```python
from build123d import *

# Parameters (mm, degrees)
EXTRUDE_1_DEPTH     = 5
EXTRUDE_7_DEPTH     = 2.220844282
CUT_EXTRUDE_5_DEPTH = 4.5
SKETCH_22_W         = 3
SKETCH_22_H         = 6
CUT_EXTRUDE_7_DEPTH = 10
SKETCH_24_W         = 3
SKETCH_24_H         = 6
CUT_EXTRUDE_8_DEPTH = 2
SKETCH_25_W         = 3
SKETCH_25_H         = 6
CUT_EXTRUDE_9_DEPTH = 2


with BuildPart() as part:
    # 草圖1 → 填料-伸長1 (new, symmetric)
    with BuildSketch(Plane.XY):
        with BuildLine():
            Line((0, 0), (0, -20))
            ThreePointArc((0, -20), (4.217076995, -21.746770485), (8.434153991, -20))
            Line((8.434153991, -20), (8.434153991, 0))
            ThreePointArc((8.434153991, 0), (4.217076995, 1.305083655), (0, 0))
        make_face()
    extrude(amount=EXTRUDE_1_DEPTH, both=True)

    # 草圖19 → 填料-伸長7 (add, symmetric)
    with BuildSketch(Plane(origin=(-5.031859453, -10, 0), x_dir=(1, 0, 0), z_dir=(0, 1, 0))):
        with BuildLine():
            Line((8.364623855, 4.848181061), (19.186976182, 4.848181061))
            ThreePointArc((19.186976182, 4.848181061), (24.038353521, -0.003196277), (19.186976182, -4.854573616))
            Line((19.186976182, -4.854573616), (8.364623855, -4.854573616))
            Line((8.364623855, -4.854573616), (8.364623855, 4.848181061))
        make_face()
    extrude(amount=EXTRUDE_7_DEPTH, both=True)

    # 草圖21 → 除料-伸長5 (cut)
    with BuildSketch(Plane(origin=(0, -7.779155718, 0), x_dir=(1, 0, 0), z_dir=(0, 1, 0))):
        with BuildLine():
            Line((8.434153991, 3.848181061), (14.041459842, 3.848181061))
            ThreePointArc((14.041459842, 3.848181061), (17.892837181, -0.003196277), (14.041459842, -3.854573616))
            Line((14.041459842, -3.854573616), (8.434153991, -3.854573616))
            Line((8.434153991, -3.854573616), (8.434153991, 3.848181061))
        make_face()
    extrude(amount=-CUT_EXTRUDE_5_DEPTH, mode=Mode.SUBTRACT)

    # 草圖22 → 除料-伸長7 (cut)
    with BuildSketch(Plane.XY.offset(5)):
        with Locations((4.5, -10.185420111)):
            Rectangle(SKETCH_22_W, SKETCH_22_H)
    extrude(amount=-CUT_EXTRUDE_7_DEPTH, mode=Mode.SUBTRACT)

    # 草圖24 → 除料-伸長8 (cut)
    with BuildSketch(Plane(origin=(0, 0, -5), x_dir=(-1, 0, 0), z_dir=(0, 0, -1))):
        with Locations((-1.5, -10.185420111)):
            Rectangle(SKETCH_24_W, SKETCH_24_H)
    extrude(amount=-CUT_EXTRUDE_8_DEPTH, mode=Mode.SUBTRACT)

    # 草圖25 → 除料-伸長9 (cut)
    with BuildSketch(Plane.XY.offset(5)):
        with Locations((1.5, -10.185420111)):
            Rectangle(SKETCH_25_W, SKETCH_25_H)
    extrude(amount=-CUT_EXTRUDE_9_DEPTH, mode=Mode.SUBTRACT)


solid = part.part
```
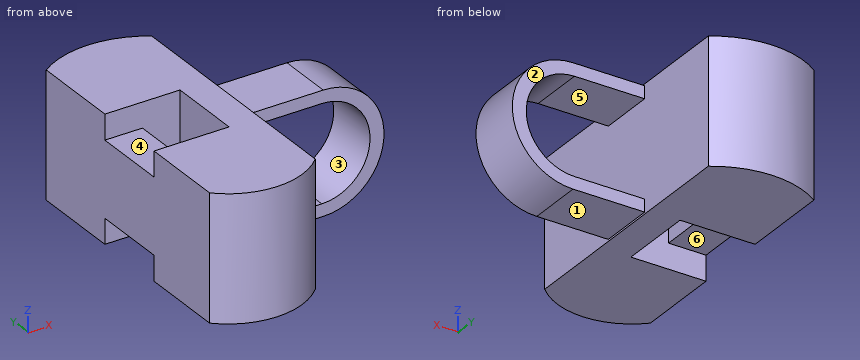
Input: part model. Units: mm. Frame: model coordinates. Face numbers are marked on the shaded views. A direction names the side the tool comes from. Coordinates: 2 decimals unless noted, no trailing zeros. Loops run counter-clockwise (first coordinate to the right, second up) from the corner with the lowest first, then second, coordinate; pieces in that order, holes last. Notation, with made-up numbers: M 83.5,-27 L 115.5,-27 A28 ccw 115.5,-4 Z; hole C 34,76.25 d9. An arc over 180 degrees is marked long. Use a Markdown table: item, result. Add a question column.
1) Set-up query: the marked faces 4, 5 and 6. Return all of +Z, -Z, +X, -X, +Y, -Y with unobstructed straight access to the full face (end or side cutting, diameter ignored); none if empty.
2) Section B-B, the plane z = 0.75. Return the cut outline in (x, y), plus the area to 3 significant figures.
3) Draft query along Z for the marked faces 1, 2 and 3. Return one class per face: +Z half, -Z half, draft (parallel to the pull), parting line (faces both ways), or undercut.
4) Line query: L1, parallel to X at y = -11.5, z = 0; L2, parallel to X at y = -10, z = -2.5; L3, parallel to Y at x = 4, z = 2.5. Output: solid intervals per line, ascending. Write a range as from..to.
5) Section C-C, the plane x = 16. Return the cut outline in (y, z), plus the area to 3 significant figures.
6) Section D-D, the plane z = -3.5. Return the cut outline in (x, y), plus the area to 3 significant figures.
7) Pin query (flat end, axial travel): P1, Ø3, axis at x = 12, z = -1, coming from the -Y side; P2, Ø5, axis at y = -13.5, z = -2.5, coming from the +X side; P3, Ø2.5, axis at x = 2, y = -11.5, coming from the +Z side; P4, Ø3.5, axis at x = 10.5, y = -9.5, coming from the -Z side. Return the tip coordinate at first contact, or that it passes through.
8) Section A-A, the plane y = -11.75. Return the cut outline in (x, z).
Answer below:
| question | item | result |
|---|---|---|
| 1 | face 4 | +Z, -X |
| 1 | face 5 | +Y, -Y |
| 1 | face 6 | -Z, -X |
| 2 | outline | M 0,-20 A5.96 ccw 8.43,-20 L 8.43,0 A7.47 ccw 0,0 Z; M 17.82,-12.22 L 18.95,-12.22 L 18.95,-7.78 L 17.82,-7.78 Z; hole M 3,-13.19 L 6,-13.19 L 6,-7.19 L 3,-7.19 Z |
| 2 | area | 173 mm2 |
| 3 | face 1 | -Z half |
| 3 | face 2 | draft |
| 3 | face 3 | undercut |
| 4 | L1 | 0..3, 6..8.43, 17.89..19.01 |
| 4 | L2 | 0..3, 6..8.43, 16.97..18.31 |
| 4 | L3 | -21.74..-13.19, -7.19..1.3 |
| 5 | outline | M -12.22,-4.48 L -7.78,-4.48 L -7.78,-3.31 L -12.22,-3.31 Z; M -12.22,3.32 L -7.78,3.32 L -7.78,4.49 L -12.22,4.49 Z |
| 5 | area | 10.4 mm2 |
| 6 | outline | M 0,-20 A5.96 ccw 8.43,-20 L 8.43,0 A7.47 ccw 0,0 L 0,-7.19 L 6,-7.19 L 6,-13.19 L 0,-13.19 Z; M 15.64,-12.22 L 17.51,-12.22 L 17.51,-7.78 L 15.64,-7.78 Z |
| 6 | area | 159 mm2 |
| 7 | P1 | through |
| 7 | P2 | x = 18.99 |
| 7 | P3 | z = 3 |
| 7 | P4 | z = -4.85 |
| 8 | outline | M 0,-3 L 3,-3 L 3,3 L 0,3 Z; M 6,-5 L 8.43,-5 L 8.43,-4.85 L 14.16,-4.85 A4.85 ccw 14.16,4.85 L 8.43,4.85 L 8.43,5 L 6,5 Z; hole M 8.43,-3.85 L 14.04,-3.85 A3.85 ccw 14.04,3.85 L 8.43,3.85 Z |
